Build history of the part. All positions in model axes, mm. A direction names the side the tool comes from. Round coordinates to 2 decimals unless told otherwise and drop trailing zeros. Write each loop counter-clockwise with the first axis right and the second up, starting at its lowest first coordinate (ties: lowest second). Pieces come first, ordered by that corner, then holes. Notation, with made-up numbers: (71, 15) -> (112, 15) arc R29 cw to (112, 41) -> close; hole circle Ø2 at (80.5, 68.25). An arc over 180 degrees is marked (long way). Answer as CSV lines item,"result".
from build123d import *

# Parameters (mm, degrees)
F1_DEPTH = 41.275
F2_R     = 10.3124
F3_DEPTH = 50.8
F5_DEPTH = 41.276


with BuildPart() as f1:
    # F0 (on Front) → F1 (new body)
    with BuildSketch(Plane.XZ):
        Polygon((0, 71.4375), (0, 0), (304.8, 0), (304.8, 15.875), align=None)
    extrude(amount=F1_DEPTH)

    # F2 (on face) → F3 (cut)
    with BuildSketch(Plane(origin=(0, 0, 0), x_dir=(0, -1, 0), z_dir=(-1, 0, 0))):
        with Locations((20.6375, 32.5501)):
            Circle(F2_R)
    extrude(amount=-F3_DEPTH, mode=Mode.SUBTRACT)

    # F4 (on face) → F5 (cut, through all)
    with BuildSketch(Plane.XZ.offset(41.275)):
        Polygon((35.428196, 0), (0, 20.679992), (0, 0), align=None)
        with BuildLine():
            ThreePointArc((138.269581, 34.907452), (174.836839, 25.4808), (209.619478, 10.777256))
            ThreePointArc((209.619478, 10.777256), (213.276315, 5.277363), (209.305078, 0))
            Line((209.305078, 0), (304.8, 0))
            Line((304.8, 0), (304.8, 15.875))
            Line((304.8, 15.875), (0, 71.4375))
            Line((0, 71.4375), (0, 58.861777))
            Line((0, 58.861777), (134.772693, 35.513265))
            ThreePointArc((134.772693, 35.513265), (136.522187, 35.216418), (138.269581, 34.907452))
        make_face()
    extrude(amount=-F5_DEPTH, mode=Mode.SUBTRACT)


solid = f1.part
1. Which spindle directions (+Z, -Z, +X, -X, +Y, -Y) get a long thin tool onto all of the face, cutting with end or side? Do faces 4 (the cylindrical face through (25.044, -30.164, 28.6)), 5 (the cylindrical face through (174.34, -20.93, 25.65)). Say none if no direction does.
Results found:
face 4,"-X"
face 5,"+Z, +X, +Y, -Y"
2. Mould opens along Y. For faces 1 (the flat face through (81, -41.275, 23)), 2 (the cylindrical face through (213.28, -20.93, 5.38)), 3 (the flat face through (50.8, -20, 33)) say: +Y half, -Y half, draft (parallel to the pull), parting line (faces both ways), or undercut.
Results found:
face 1,"-Y half"
face 2,"draft"
face 3,"undercut"
3. Probe line 1 along Y through (x, z) = (48, 34) (3 decimals); line 2 along Y through (x, z) = (45, 37) (3 decimals); line 3 along Z through (x, y) = (42, -15). List the from-to ranges inside material, lowest first.
Results found:
line 1,"y = -41.275 to -30.847, -10.428 to 0"
line 2,"y = -41.275 to -29.94, -11.335 to 0"
line 3,"z = 0 to 23.92, 41.19 to 51.59"
4. Cut at D-D, the plane x = 156.5. Write the cut outline in (y, z) (3 decimals).
Results found:
outline,"(-41.275, 0) -> (0, 0) -> (0, 30.928) -> (-41.275, 30.928) -> close"
5. Cut at C-C, the plane z = 41. Write the cut outline in (x, y) (3 decimals), then the cut area to 3 significant figures.
Results found:
outline,"(0, -41.275) -> (103.102, -41.275) -> (103.102, 0) -> (0, 0) -> (0, -14.726) -> (50.8, -14.726) -> (50.8, -26.549) -> (0, -26.549) -> close"
area,"3,650 mm2"
6. Drop flat-ended pins along their axis: pin 1 Ø12 at (y, z) = (-18.5, 24.5) entering from +X; pin 2 Ø8 at (x, y) = (145.5, -32.5) entering from +Z; pin 3 Ø2 at (x, y) = (134, -12.5) entering from +Z; pin 4 Ø8 at (y, z) = (-28, 22.5) entering from -X. Give the stop position or say it passes through.
Results found:
pin 1,"stops at x = 193.14"
pin 2,"stops at z = 34.3"
pin 3,"stops at z = 35.82"
pin 4,"stops at x = 0"
7. Cut at A-A, the plane y = -36. Write the cut outline in (x, z).
Results found:
outline,"(0, 20.68) -> (35.43, 0) -> (209.31, 0) arc R5.72 ccw to (209.62, 10.78) arc R256 ccw to (138.27, 34.91) arc R256.01 ccw to (134.77, 35.51) -> (0, 58.86) -> close"
8. Cut at B-B, the plane x = 46. Write the cut outline in (y, z) (1 decimal), then the cut area to 3 significant figures.
Results found:
outline,"(-41.3, 0) -> (0, 0) -> (0, 50.9) -> (-41.3, 50.9) -> close; hole circle Ø20.6 at (-20.6, 32.6)"
area,"1,770 mm2"
